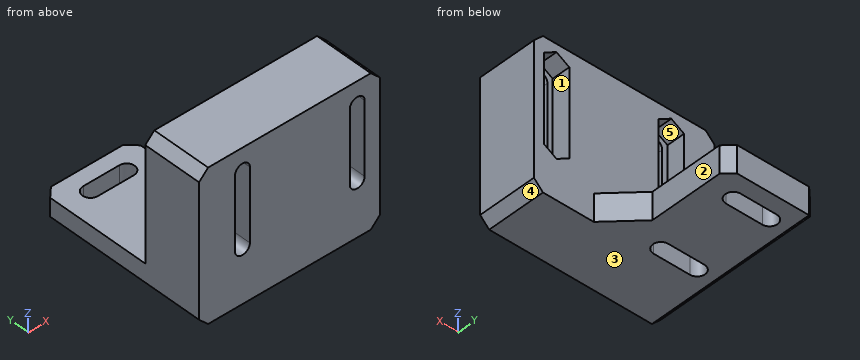
Autodesk Inventor part; units mm, degrees
ref_plane "YZ Plane" through (0, 0, 0) normal (1, 0, 0) x (0, 1, 0)
ref_plane "XZ Plane" through (0, 0, 0) normal (0, 1, 0) x (-1, 0, 0)
ref_plane "XY Plane" through (0, 0, 0) normal (0, 0, 1) x (1, 0, 0)
sketch "Sketch1" plane through (0, 0, 0) normal (1, 0, 0) x (0, 1, 0)
  line L0 (0, 0) -> (13, 0)
  line L1 (13, 0) -> (13, -27)
  line L2 (13, -27) -> (0, -27)
  line L3 (0, -27) -> (0, 0)
  dimension "d0" = 13
  dimension "d1" = 27
extrude "Extrusion1" add sketch "Sketch1" along normal blind 40
sketch "Sketch2" plane through (40, 0, 0) normal (1, 0, 0) x (0, 0, -1)
  line L0 (27, 0) -> (27, 13)
  line L1 (27, 0) -> (33, 0)
  line L2 (33, 0) -> (33, 38)
  line L3 (33, 38) -> (27, 38)
  line L4 (27, 38) -> (27, 0)
  point P0 (0, 0)
  dimension "d4" = 6
  dimension "d5" = 38
extrude "Extrusion2" add sketch "Sketch2" against normal blind 40
sketch "Sketch3" plane through (0, 13, 0) normal (0, 1, 0) x (1, 0, 0)
  line L0 (40, 27) -> (40, 0) construction
  line L1 (40, 0) -> (35, 0) construction
  line L2 (0, 0) -> (40, 0) construction
  line L3 (35, 0) -> (35, 5) construction
  line L4 (35, 5) -> (35, 21) construction
  line L5 (35, 5) -> (9.6, 5) construction
  line L6 (35, 5) -> (35, 21) construction
  line L7 (36.65, 5) -> (36.65, 21)
  line L8 (33.35, 21) -> (33.35, 5)
  arc A0 (33.35, 5) -> (36.65, 5) centre (35, 5) ccw
  arc A1 (36.65, 21) -> (33.35, 21) centre (35, 21) ccw
  line L9 (9.6, 0) -> (9.6, 5) construction
  line L10 (9.6, 5) -> (9.6, 21) construction
  line L11 (9.6, 5) -> (-15.8, 5) construction
  line L12 (9.6, 5) -> (9.6, 21) construction
  line L13 (11.25, 5) -> (11.25, 21)
  line L14 (7.95, 21) -> (7.95, 5)
  arc A2 (7.95, 5) -> (11.25, 5) centre (9.6, 5) ccw
  arc A3 (11.25, 21) -> (7.95, 21) centre (9.6, 21) ccw
  point P0 (35, 13)
  point P1 (9.6, 13)
  dimension "d8" = 5
  dimension "d9" = 5
  dimension "d10" = 16
  dimension "d11" = 25.4
  dimension "d12" = 3.3
  dimension "d13" = 5
  dimension "d14" = 16
  dimension "d15" = 25.4
  dimension "d16" = 3.3
extrude "Extrusion3" cut sketch "Sketch3" against normal blind 40
sketch "Sketch4" plane through (0, 13, 0) normal (0, 1, 0) x (1, 0, 0)
  point P0 (0, 0)
sketch "Sketch5" plane through (0, 13, 0) normal (0, 1, 0) x (1, 0, 0)
  arc A0 (33.35, 5) -> (36.65, 5) centre (35, 5) ccw
  line L0 (35, 5) -> (32.1806, 5) construction
  line L1 (35, 5) -> (37.8194, 5) construction
  line L2 (37.8194, 6.6278) -> (37.8194, 3.3722)
  line L3 (37.8194, 3.3722) -> (35, 1.7444)
  line L4 (35, 1.7444) -> (32.1806, 3.3722)
  line L5 (32.1806, 3.3722) -> (32.1806, 6.6278)
  arc A1 (36.65, 21) -> (33.35, 21) centre (35, 21) ccw
  line L6 (35, 21) -> (32.1806, 21) construction
  line L7 (32.1806, 22.6278) -> (35, 24.2556)
  line L8 (35, 24.2556) -> (37.8194, 22.6278)
  line L9 (37.8194, 22.6278) -> (37.8194, 19.3722)
  line L10 (32.1806, 19.3722) -> (32.1806, 22.6278)
  line L11 (32.1806, 19.3722) -> (32.1806, 6.6278)
  line L12 (33.35, 5) -> (33.35, 21)
  line L13 (36.65, 5) -> (36.65, 21)
  line L14 (37.8194, 19.3722) -> (37.8194, 6.6278)
  arc A2 (7.95, 5) -> (11.25, 5) centre (9.6, 5) ccw
  line L15 (9.6, 5) -> (6.7806, 5) construction
  line L16 (9.6, 5) -> (12.4194, 5) construction
  line L17 (12.4194, 6.6278) -> (12.4194, 3.3722)
  line L18 (12.4194, 3.3722) -> (9.6, 1.7444)
  line L19 (9.6, 1.7444) -> (6.7806, 3.3722)
  line L20 (6.7806, 3.3722) -> (6.7806, 6.6278)
  line L21 (9.6, 21) -> (6.7806, 21) construction
  line L22 (6.7806, 22.6278) -> (9.6, 24.2556)
  line L23 (9.6, 24.2556) -> (12.4194, 22.6278)
  line L24 (12.4194, 22.6278) -> (12.4194, 19.3722)
  line L25 (6.7806, 19.3722) -> (6.7806, 22.6278)
  line L26 (6.7806, 19.3722) -> (6.7806, 6.6278)
  line L27 (12.4194, 19.3722) -> (12.4194, 6.6278)
  point P0 (0, 0)
  dimension "d19" = 2.8194
  dimension "d20" = 2.8194
  dimension "d21" = 2.8194
  dimension "d23" = 2.8194
  dimension "d24" = 2.8194
  dimension "d25" = 2.8194
extrude "Extrusion4" cut sketch "Sketch5" against normal blind 4 contours L12 A1 L13 A0 | L2 L3 L4 L5 L11 L10 L7 L8 L9 L14 | L17 L18 L19 L20 L26 L25 L22 L23 L24 L27
sketch "Sketch6" plane through (40, 13, -27) normal (0, 0, 1) x (1, 0, 0)
  line L0 (-40, 0) -> (0, 0) construction
  line L1 (-40, 0) -> (-40, 2.3) construction
  line L2 (-40, 25) -> (-40, -13) construction
  line L3 (-40, 2.3) -> (-6.5941, 2.3) construction
  line L4 (-40, 2.3) -> (-40, 19.8) construction
  line L5 (-40, 19.8) -> (-7.5372, 19.8) construction
  line L6 (-40, 2.3) -> (-34, 2.3) construction
  line L7 (-34, 2.3) -> (-34, 19.8) construction
  line L8 (-34, 19.8) -> (-26, 19.8) construction
  line L9 (-34, 2.3) -> (-26, 2.3) construction
  line L10 (-34, 19.8) -> (-26, 19.8) construction
  line L11 (-34, 18.05) -> (-26, 18.05)
  line L12 (-26, 21.55) -> (-34, 21.55)
  arc A0 (-34, 21.55) -> (-34, 18.05) centre (-34, 19.8) ccw
  arc A1 (-26, 18.05) -> (-26, 21.55) centre (-26, 19.8) ccw
  line L13 (-34, 2.3) -> (-26, 2.3) construction
  line L14 (-34, 0.55) -> (-26, 0.55)
  line L15 (-26, 4.05) -> (-34, 4.05)
  arc A2 (-34, 4.05) -> (-34, 0.55) centre (-34, 2.3) ccw
  arc A3 (-26, 0.55) -> (-26, 4.05) centre (-26, 2.3) ccw
  point P0 (-30, 19.8)
  point P1 (-30, 2.3)
  dimension "d28" = 2.3
  dimension "d29" = 17.5
  dimension "d30" = 6
  dimension "d31" = 8
  dimension "d32" = 8
  dimension "d33" = 3.5
  dimension "d34" = 3.5
extrude "Extrusion5" cut sketch "Sketch6" against normal blind 35.6875
sketch "Sketch7" plane through (40, 13, -27) normal (0, 0, 1) x (1, 0, 0)
  line L0 (0, 25) -> (0, 0)
  line L1 (-40, 0) -> (0, 0)
  line L2 (0, 25) -> (-20, 25)
  line L3 (-20, 25) -> (-20, 0)
  line L4 (-20, 0) -> (0, 0)
  line L5 (0, 0) -> (0, 25)
  point P0 (-40, -13)
extrude "Extrusion6" cut sketch "Sketch7" against normal blind 45.275
chamfer "Chamfer1" distance 6.7625 angle 45 1 edges at (20, 13, -30)
chamfer "Chamfer2" distance 2 angle 45 1 edges at (20, 38, -30)
chamfer "Chamfer3" distance 2 angle 45 1 edges at (0, 38, -30)
chamfer "Chamfer4" distance 2 angle 45 4 edges at (40, 6.5, 0) (0, 6.5, 0) (40, 6.5, -33) (0, 18, -33)
sketch "Sketch8" plane through (0, 13, -27) normal (0, 1, 0) x (1, 0, 0)
  line L0 (0, 0) -> (26.7625, 0) construction
  line L1 (0, 0) -> (2.5, 0) construction
  line L2 (2.5, 0) -> (14.5, 0)
  line L3 (14.5, 0) -> (14.5, -7)
  line L4 (14.5, -7) -> (2.5, -7)
  line L5 (2.5, -7) -> (2.5, 0)
  point P0 (0, -27)
  dimension "d53" = 2.5
  dimension "d54" = 12
  dimension "d55" = 7
extrude "Extrusion7" cut sketch "Sketch8" against normal blind 1.5
properties part number "Motor Mount"
For this review, take the finished solid that the model builds, in its own axes (mm). Face numbers are marked on the shaded views. A direction names the side the tool comes from. Give positions to 0.01 mm unless a question says otherwise; leave off trailing zeros. Write each loop counter-clockwise with the first axis right and the second up, starting at its lowest first coordinate (ties: lowest second). Pieces come first, ordered by that corner, then holes. Notation, with made-up numbers: M 52.25,-25.75 L 58.25,-25.75 A11 cw 58.25,-9.75 Z; hole C 33.25,-19.75 d8. An arc over 180 degrees is marked long. Answer as a JSON object with one key per item and string values. Group by question number.
Item 1: For pin 1 Ø10 at (x, z) = (23, -9) entering from +Y; pin 2 Ø1.5 at (x, z) = (23.5, -29.5) entering from -Y; pin 3 Ø4.5 at (x, z) = (9.5, -15.5) entering from +Y; pin 4 Ø6.5 at (y, z) = (28.5, -31.5) entering from +X, all flat-tipped, find the tip position at first contact; note any pin that passes through.
Item 2: Consider section D-D on z = -29.5. Write out the cut boundary in (x, y), plus the area to 3 significant figures.
Item 3: Consider section C-C on y = 7. Write out the cut boundary in (x, z).
Item 4: Tool access review of the marked faces 4 and 5: name each direction out of +Z, -Z, +X, -X, +Y, -Y from which nothing blocks a thin tool from reaching the whole face with its end or side.
Item 5: For probe 1 along X at (y, z) = (12.5, -21); probe 2 along X at (y, z) = (2.5, -9); probe 3 along Y at (x, z) = (11.5, -28.5), list the stretches that pass through material, from the lowest coordinate up. Write a range as [from, to].
Item 6: Consider section A-A on z = -15. Write out the cut boundary in (x, y).
Item 7: Consider section B-B on y = 32.8. Write out the cut boundary in (x, z).
Item 8: Draft analysis for pull direction X (two halves, no side actions). For the marked faces 1, 2 and 3, state which applies: +X half, -X half, draft (parallel to the pull), parting line (faces both ways), or undercut.
Check result:
{
 "1": {"pin 1": "stops at y = 13", "pin 2": "stops at y = 0", "pin 3": "stops at y = 9", "pin 4": "stops at x = 20"},
 "2": {"outline": "M 0,0 L 40,0 L 40,13 L 26.76,13 L 20,19.76 L 20,36 L 18,38 L 2,38 L 0,36 Z; hole M 6,13.55 L 14,13.55 A1.75 ccw 14,17.05 L 6,17.05 A1.75 ccw Z; hole M 6,31.05 L 14,31.05 A1.75 ccw 14,34.55 L 6,34.55 A1.75 ccw Z", "area": "964 mm^2"},
 "3": {"outline": "M 0,-31 L 2,-33 L 38,-33 L 40,-31 L 40,-2 L 38,0 L 2,0 L 0,-2 Z; hole M 7.95,-21 A1.65 ccw 11.25,-21 L 11.25,-5 A1.65 ccw 7.95,-5 Z; hole M 33.35,-21 A1.65 ccw 36.65,-21 L 36.65,-5 A1.65 ccw 33.35,-5 Z"},
 "4": {"face 4": "-Z, +X, +Y, -Y", "face 5": "+Y"},
 "5": {"probe 1": "x = [0, 2.5], [14.5, 32.18], [37.82, 40]", "probe 2": "x = [0, 7.95], [11.25, 33.35], [36.65, 40]", "probe 3": "y = [0, 13.55], [17.05, 31.05], [34.55, 38]"},
 "6": {"outline": "M 0,0 L 7.95,0 L 7.95,9 L 6.78,9 L 6.78,13 L 0,13 Z; M 11.25,0 L 33.35,0 L 33.35,9 L 32.18,9 L 32.18,13 L 12.42,13 L 12.42,9 L 11.25,9 Z; M 36.65,0 L 40,0 L 40,13 L 37.82,13 L 37.82,9 L 36.65,9 Z"},
 "7": {"outline": "M 0,-31 L 2,-33 L 4.25,-33 L 4.25,-27 L 0,-27 Z; M 15.75,-33 L 20,-33 L 20,-27 L 15.75,-27 Z"},
 "8": {"face 1": "undercut", "face 2": "+X half", "face 3": "draft"}
}
